```python
from build123d import *

# Parameters (mm, degrees)
ESBO_O1_R                = 5.35
ESBO_O1_R_2              = 1.75
RESSALTO_EXTRUS_O1_DEPTH = 10
ESBO_O2_R                = 1.75
CORTE_EXTRUS_O1_DEPTH    = 10


with BuildPart() as part:
    # Esboço1 → Ressalto-extrusão1 (new body)
    with BuildSketch(Plane.XY):
        Polygon((-11, -5), (-11, -15), (11, -15), (11, -5), (20, -5), (20, 0), (-20, 0), (-20, -5), align=None)
        with Locations((0, -6.75)):
            Circle(ESBO_O1_R, mode=Mode.SUBTRACT)
        with Locations((-8, -6.75)):
            Circle(ESBO_O1_R_2, mode=Mode.SUBTRACT)
        with Locations((8, -6.75)):
            Circle(ESBO_O1_R_2, mode=Mode.SUBTRACT)
    extrude(amount=RESSALTO_EXTRUS_O1_DEPTH)

    # Esboço2 → Corte-extrusão1 (cut)
    with BuildSketch(Plane(origin=(0, 0, 0), x_dir=(1, 0, 0), z_dir=(0, 1, 0))):
        with Locations(Location((-15, -5, 0), (0, 0, 180))):
            Circle(ESBO_O2_R)
        with Locations(Location((15, -5, 0), (0, 0, 180))):
            Circle(ESBO_O2_R)
    extrude(amount=-CORTE_EXTRUS_O1_DEPTH, mode=Mode.SUBTRACT)


solid = part.part
```
Source: CAD feature listing. Evaluate the final solid. Frame: model axes, mm. A direction names the side the tool comes from. Coordinates: 2 decimals unless noted, no trailing zeros. Order: outer loops, then holes, each group sorted by start corner. A loop starts at its lowest first (then second) coordinate and runs counter-clockwise, first axis right, second up. Notation, with made-up numbers: (7, 57) - (20, 57) arc R33 ccw to (20, 92) - close; hole circle Ø9 at (71.5, 41). An arc over 180 degrees is marked (long way). One line per item, written item: value.
1) Reachability of faces 1 (the face through (17, -5, 5)), 2 (the face through (-11, -10, 5)), 3 (the face through (-7.19, -8.3, 4.93)) from +Z, -Z, +X, -X, +Y, -Y: full face, straight path, thin tool, end or side. Return the list, or none.
Computed values:
face 1: +Z, -Z, +X, -Y
face 2: +Z, -Z, -X, -Y
face 3: +Z, -Z
2) Cut plane A-A on y = -6.75. Output: boundary loops of the cut face in (x, z), plus the area to 3 significant figures.
Computed values:
outline: (-11, 0) - (-9.75, 0) - (-9.75, 10) - (-11, 10) - close; (-6.25, 0) - (-5.35, 0) - (-5.35, 10) - (-6.25, 10) - close; (5.35, 0) - (6.25, 0) - (6.25, 10) - (5.35, 10) - close; (9.75, 0) - (11, 0) - (11, 10) - (9.75, 10) - close
area: 43.0 mm^2
3) Mould query, pull axis Z, two halves, no side actions, for faces 4 (the face through (-17, -5, 4)), 5 (the face through (-15.81, -2.46, 3.45)), 6 (the face through (-5, -4, 10)), 7 (the face through (14.19, -2.46, 3.45)). Classes: released by +Z, released by -Z, zero draft, split by the parting line, or undercut.
Computed values:
face 4: zero draft
face 5: undercut
face 6: released by +Z
face 7: undercut
4) Cut plane C-C on x = 0. Output: boundary loops of the cut face in (y, z), plus the area to 3 significant figures.
Computed values:
outline: (-15, 0) - (-12.1, 0) - (-12.1, 10) - (-15, 10) - close; (-1.4, 0) - (0, 0) - (0, 10) - (-1.4, 10) - close
area: 43.0 mm^2
5) Cut plane D-D on y = -4.25. Output: boundary loops of the cut face in (x, z).
Computed values:
outline: (-20, 0) - (-4.73, 0) - (-4.73, 10) - (-20, 10) - close; (4.73, 0) - (20, 0) - (20, 10) - (4.73, 10) - close; hole circle Ø3.5 at (-15, 5); hole circle Ø3.5 at (15, 5)
6) Contact query for flat-ended pins moving along their axis: pin 1 (1.5 mm diameter, centred on x = 14.5, z = 3, fed in from -Y); pin 2 (6 mm diameter, centred on y = -9.5, z = 2, fed in from +X); pin 3 (3 mm diameter, centred on x = -15, z = 5, fed in from -Y); pin 4 (1 mm diameter, centred on y = -12, z = 9, fed in from -X). Output: stop coordinate, or through.
Computed values:
pin 1: stops at y = -5
pin 2: stops at x = 11
pin 3: passes through
pin 4: stops at x = -11
7) Ray query, line 1 (Y direction, x = -8, z = 5); line 2 (Z direction, x = 15, y = -3); line 3 (X direction, y = -0.5, z = 3.5). Return the intervals inside material, ascending. Write a range as [from, to].
Computed values:
line 1: y = [-15, -8.5], [-5, 0]
line 2: z = [0, 3.25], [6.75, 10]
line 3: x = [-20, -15.9], [-14.1, 14.1], [15.9, 20]
8) Cut plane B-B on z = 7.5. Output: boundary loops of the cut face in (x, y), plus the area to 3 significant figures.
Computed values:
outline: (-20, -5) - (-11, -5) - (-11, -15) - (11, -15) - (11, -5) - (20, -5) - (20, 0) - (-20, 0) - close; hole circle Ø3.5 at (-8, -6.75); hole circle Ø10.7 at (0, -6.75); hole circle Ø3.5 at (8, -6.75)
area: 311 mm^2
